Read the model definition and answer for the solid it produces. Units are mm, in the model's axes. Face numbers are marked on the shaded views. A direction names the side the tool comes from. Coordinates: 2 decimals unless noted, no trailing zeros. Loops run counter-clockwise (first coordinate to the right, second up) from the corner with the lowest first, then second, coordinate; pieces in that order, holes last. Notation, with made-up numbers: (-22.75, 30.25) - (15.25, 30.25) arc R9 cw to (15.25, 36.25) - close; hole circle Ø10 at (27.25, 54). An arc over 180 degrees is marked (long way). One line per question, with ' | ' between items. Start each with the question number.
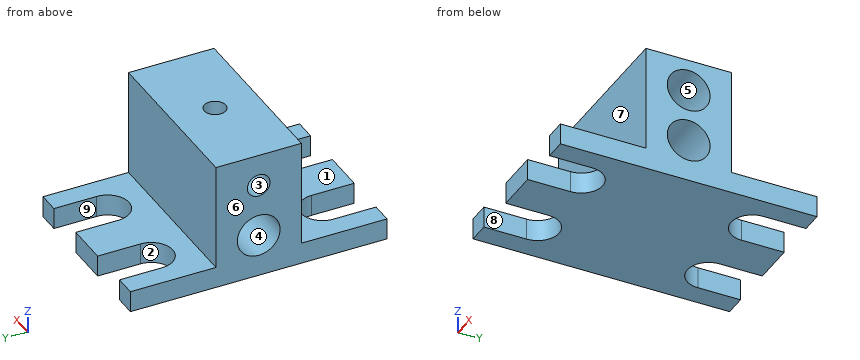
```python
from build123d import *

# Parameters (mm, degrees)
SKETCH_R         = 3.175
PAD_DEPTH        = 25.4
SKETCH001_R      = 1.5875
POCKET_DEPTH     = 4.7625
HOLE_D           = 3.18262
HOLE_DEPTH       = 14.2875
HOLE_CBORE_D     = 6.35
HOLE_CBORE_DEPTH = 10.16
POCKET001_DEPTH  = 5
SKETCH004_R      = 1.6859
HOLE001_DEPTH    = 8.89


with BuildPart() as part:
    # Sketch → Pad (new body)
    with BuildSketch(Plane.YZ):
        Polygon((-19.05, 0), (19.05, 0), (19.05, 3.175), (6.35, 3.175), (6.35, 19.05), (-6.35, 19.05), (-6.35, 3.175), (-19.05, 3.175), align=None)
        with Locations((0, 6.35)):
            Circle(SKETCH_R, mode=Mode.SUBTRACT)
    extrude(amount=PAD_DEPTH)

    # Sketch001 (on Face5 of Pad) → Pocket (cut)
    with BuildSketch(Plane(origin=(0, 0, 19.05), x_dir=(0, -1, 0), z_dir=(0, 0, 1))):
        with Locations((0, 12.7)):
            Circle(SKETCH001_R)
    extrude(amount=-POCKET_DEPTH, mode=Mode.SUBTRACT)

    # Hole
    with Locations(Plane.YZ.offset(25.4)):
        with Locations((0, 14.2875)):
            CounterBoreHole(HOLE_D / 2, HOLE_CBORE_D / 2, HOLE_CBORE_DEPTH, depth=HOLE_DEPTH)

    # Sketch003 (on Face7 of Hole) → Pocket001 (cut)
    with BuildSketch(Plane(origin=(0, 0, 3.175), x_dir=(0, -1, 0), z_dir=(0, 0, 1))):
        with BuildLine():
            Line((25.4, 9.525), (12.7, 9.525))
            ThreePointArc((12.7, 9.525), (9.525, 6.35), (12.7, 3.175))
            Line((12.7, 3.175), (25.4, 3.175))
            Line((25.4, 3.175), (25.4, 9.525))
        make_face()
        with BuildLine():
            Line((25.4, 22.225), (12.7, 22.225))
            ThreePointArc((12.7, 22.225), (9.525, 19.05), (12.7, 15.875))
            Line((12.7, 15.875), (25.4, 15.875))
            Line((25.4, 15.875), (25.4, 22.225))
        make_face()
        with BuildLine():
            Line((-25.4, 22.225), (-12.7, 22.225))
            ThreePointArc((-12.7, 15.875), (-9.525, 19.05), (-12.7, 22.225))
            Line((-12.7, 15.875), (-25.4, 15.875))
            Line((-25.4, 15.875), (-25.4, 22.225))
        make_face()
        with BuildLine():
            Line((-25.4, 9.525), (-12.7, 9.525))
            ThreePointArc((-12.7, 3.175), (-9.525, 6.35), (-12.7, 9.525))
            Line((-12.7, 3.175), (-25.4, 3.175))
            Line((-25.4, 3.175), (-25.4, 9.525))
        make_face()
    extrude(amount=-POCKET001_DEPTH, mode=Mode.SUBTRACT)

    # Sketch004 (on Face2 of Pocket001) → Hole001 (cut)
    with BuildSketch(Plane(origin=(0, 0, 0), x_dir=(0, 1, 0), z_dir=(-1, 0, 0))):
        with Locations((0, -14.2875)):
            Circle(SKETCH004_R)
    extrude(amount=-HOLE001_DEPTH, mode=Mode.SUBTRACT)


solid = part.part
```
1) Find the intervals of material crossed by line 1 along X through (y, z) = (-15.5, 1.75) (3 decimals); line 2 along Z through (x, y) = (2, 0) (3 decimals); line 3 along Z through (x, y) = (13.7, 0) (3 decimals), in increasing order. Write a range as from..to.
2) The mould has two halves that part along Y. Classify the marked faces 1, 2, 3 and 4: released by +Y, released by -Y, zero draft, split by the parting line, or undercut.
3) Which of the six approach directions +Z, -Z, +X, -X, +Y, -Y give full straight-line access (tool end or side, diameter ignored) to the marked faces 5, 6, 7, 8 and 9?
4) The part is cut by section D-D on x = 10. Write down the section's boundary in (y, z) (3 decimals).
5) The part is cut by section B-B on z = 6.35. Write down the section's boundary in (x, y) (3 decimals), and give its area (3 significant figures).
6) Given pin 1 Ø10 at (x, y) = (9, 14.5) entering from +Z (3 decimals); pin 2 Ø1 at (x, y) = (15, 7) entering from -Z; pin 3 Ø2.5 at (y, z) = (0, 14.5) entering from +X; pin 4 Ø5 at (x, z) = (15.5, 6.5) entering from +Y, each flat-ended and moving along its own axis, determine where each tip first touches the part or whether it passes through.
7) The part is cut by section A-A on x = 19.05. Count the separate pieces of the cut face and the enclosed holes in it, and give its area (3 significant figures).
8) The part is cut by section C-C on y = 16. Write down the section's boundary in (x, z) (3 decimals), and give its area (3 significant figures).
Answer below:
1) line 1: 0..3.175, 9.525..15.875, 22.225..25.4 | line 2: 0..3.175, 9.525..12.602, 15.973..19.05 | line 3: 0..3.175, 9.525..12.696
2) face 1: zero draft | face 2: released by +Y | face 3: undercut | face 4: undercut
3) face 5: +X | face 6: +Z, -Z, -X, +Y, -Y | face 7: +Z, +X, -X, -Y | face 8: +Z, -Z, -Y | face 9: +Z, -Z, +Y
4) outline: (-19.05, 0) - (19.05, 0) - (19.05, 3.175) - (6.35, 3.175) - (6.35, 19.05) - (-6.35, 19.05) - (-6.35, 3.175) - (-19.05, 3.175) - close; hole circle Ø6.35 at (0, 6.35)
5) outline: (0, -6.35) - (25.4, -6.35) - (25.4, -3.175) - (0, -3.175) - close; (0, 3.175) - (25.4, 3.175) - (25.4, 6.35) - (0, 6.35) - close | area: 161 mm2
6) pin 1: z = 3.175 | pin 2: z = 0 | pin 3: x = 11.11 | pin 4: y = 6.35
7) separate pieces: 1 | enclosed holes: 2 | area: 199 mm2
8) outline: (0, 0) - (3.175, 0) - (3.175, 3.175) - (0, 3.175) - close; (9.525, 0) - (15.875, 0) - (15.875, 3.175) - (9.525, 3.175) - close; (22.225, 0) - (25.4, 0) - (25.4, 3.175) - (22.225, 3.175) - close | area: 40.3 mm2
